CAD build for the part. Positions are in the model's coordinates, mm. A direction names the side the tool comes from. Give positions to 0.01 mm unless a question says otherwise; leave off trailing zeros. Loops run counter-clockwise (first coordinate to the right, second up) from the corner with the lowest first, then second, coordinate; pieces in that order, holes last.
Item 1: Drop flat-ended pins along their axis: P1, Ø2, axis at y = 11.5, z = 5.5, coming from the +X side; P2, Ø6.5, axis at x = -16.5, y = 2.5, coming from the +Z side; P3, Ø1, axis at y = 2, z = 10.5, coming from the +X side; P4, Ø9, axis at x = 18, y = 0, coming from the -Z side. Give the stop position or say it passes through.
Item 2: Saw through at C-C on x = 18. Give the cut face in (y, z), plus the area to 3 significant figures.
Item 3: Saw through at A-A on y = 0. Give the number of separate pieces and of enclosed holes in the cut face, plus the area to 3 significant figures.
Item 4: Saw through at B-B on x = 0. Give the cut face in (y, z).
Item 5: Which spindle directions (+Z, -Z, +X, -X, +Y, -Y) get a long thin tool onto all of the face, cutting with end or side? Do faces 1 (the flat face through (7.02, 8.9, 5.33)), 2 (the flat face through (-5.5, 11, 6)), 3 (the cylindrical face through (20.747, 0.121, 3.328)). Say none if no direction does.
Item 6: Probe probe 1 along X at (y, z) = (0, 4); probe 2 along Z at (x, y) = (-6.6, 10.5); probe 3 along Y at (x, z) = (8, 5.5). List the from-to ranges inside material, lowest first.
Item 7: Mould opens along Y. For faces 4 (the flat face through (7.02, 10.29, 8.47)), 5 (the flat face through (-16.32, -5.74, 3.7)), 6 (the flat face through (23.5, 0, 3)), 7 (the flat face through (7.021, 8.689, 7.304)) say: released by +Y, released by -Y, zero draft, split by the parting line, or undercut.
from build123d import *

# Parameters (mm, degrees)
BOSS_EXTRUDE1_DEPTH                                 = 13
CUT_EXTRUDE1_DEPTH                                  = 24.780243901
CUT_EXTRUDE1_DEPTH_BACK                             = 24.780243901
FILLET1_R                                           = 2
BOSS_EXTRUDE2_DEPTH                                 = 7
F_5_5_5_5_DIAMETER_HOLE1_D                          = 5.5
F_5_5_5_5_DIAMETER_HOLE1_DEPTH                      = 10
F_5_5_5_5_DIAMETER_HOLE1_CSINK_D                    = 6
F_5_5_5_5_DIAMETER_HOLE1_CSINK_ANGLE                = 90
F_5_5_5_5_DIAMETER_HOLE1_TIP                        = 1.652366702
CUT_EXTRUDE2_REACH                                  = 39.017
CBORE_FOR_M4_HEX_SOCKET_HEAD_CAP_SCREW3_D           = 3.4
CBORE_FOR_M4_HEX_SOCKET_HEAD_CAP_SCREW3_CBORE_D     = 7.5
CBORE_FOR_M4_HEX_SOCKET_HEAD_CAP_SCREW3_CBORE_DEPTH = 3
CHAMFER1_SIZE                                       = 0.2
CUT_EXTRUDE3_DEPTH                                  = 3
CHAMFER2_SIZE                                       = 0.5
FILLET2_R                                           = 0.8
CHAMFER3_SIZE                                       = 0.2
CHAMFER3_SIZE2                                      = 0.346410162


with BuildPart() as part:
    # Sketch1 → Boss-Extrude1 (new body)
    with BuildSketch(Plane.XY):
        with BuildLine():
            Line((0.75, 5.95294045), (0.75, 15.5))
            Line((0.75, 15.5), (7.5, 15.5))
            Line((7.5, 15.5), (7.5, 10))
            ThreePointArc((7.5, 10), (0, -12.5), (-7.5, 10))
            Line((-7.5, 10), (-7.5, 15.5))
            Line((-7.5, 15.5), (-0.75, 15.5))
            Line((-0.75, 15.5), (-0.75, 5.95294045))
            ThreePointArc((-0.75, 5.95294045), (0, -6), (0.75, 5.95294045))
        make_face()
    extrude(amount=BOSS_EXTRUDE1_DEPTH)

    # Sketch2 → Cut-Extrude1 (cut, two sides: drawn at the far end of the back side and taken through both)
    with BuildSketch(Plane(origin=(0, 0, 0), x_dir=(0, 0, -1), z_dir=(1, 0, 0)).offset(-CUT_EXTRUDE1_DEPTH_BACK)):
        with BuildLine():
            Line((69.410215856, 1.772448509), (0, 14.891132578))
            ThreePointArc((0, 14.891132578), (-6.5, 15.5), (-13, 14.891132578))
            Line((-13, 14.891132578), (-82.410215856, 1.772448509))
            Line((-82.410215856, 1.772448509), (-82.410215856, 143.050584636))
            Line((-82.410215856, 143.050584636), (69.410215856, 143.050584636))
            Line((69.410215856, 143.050584636), (69.410215856, 1.772448509))
        make_face()
    extrude(amount=CUT_EXTRUDE1_DEPTH + CUT_EXTRUDE1_DEPTH_BACK, mode=Mode.SUBTRACT)

    # Fillet1
    fillet1_edges = [part.edges().sort_by_distance(p)[0] for p in [
        (7.5, 10, 6.5),
        (-7.5, 10, 6.5),
    ]]
    fillet(fillet1_edges, radius=FILLET1_R)

    # Sketch3 → Boss-Extrude2 (add)
    with BuildSketch(Plane.XY):
        with BuildLine():
            Line((8.803538255, 8.873990883), (23.5, 2.75))
            Line((23.5, 2.75), (23.5, -2.75))
            Line((23.5, -2.75), (8.803538255, -8.873990883))
            ThreePointArc((8.803538255, -8.873990883), (12.5, 0), (8.803538255, 8.873990883))
        make_face()
    extrude(amount=BOSS_EXTRUDE2_DEPTH)

    # Mirror1: part across plane


with BuildPart() as part_1:
    add(part.part)
    add(part.part.mirror(Plane(origin=(0, 0, 0), x_dir=(0, 0, 1), z_dir=(1, 0, 0))))

    # Ø5.5 (5.5) Diameter Hole1
    with Locations(Plane.XY.offset(7)):
        with Locations((18, 0), (-18, 0)):
            CounterSinkHole(F_5_5_5_5_DIAMETER_HOLE1_D / 2, F_5_5_5_5_DIAMETER_HOLE1_CSINK_D / 2, depth=F_5_5_5_5_DIAMETER_HOLE1_DEPTH, counter_sink_angle=F_5_5_5_5_DIAMETER_HOLE1_CSINK_ANGLE)
            with Locations((0, 0, -(F_5_5_5_5_DIAMETER_HOLE1_DEPTH + F_5_5_5_5_DIAMETER_HOLE1_TIP / 2))):  # 118° drill point
                Cone(0, F_5_5_5_5_DIAMETER_HOLE1_D / 2, F_5_5_5_5_DIAMETER_HOLE1_TIP, mode=Mode.SUBTRACT)

    # Sketch9 → Cut-Extrude2 (cut, up to next)
    with BuildSketch(Plane(origin=(7.5, 0, 0), x_dir=(0, 0, -1), z_dir=(1, 0, 0)), mode=Mode.PRIVATE) as cut_extrude2_sk1:
        with BuildLine():
            Line((-2.023006126, 10.95445115), (-13, 10.95445115))
            Line((-13, 10.95445115), (-13, 6))
            Line((-13, 6), (-6.5, 6))
            ThreePointArc((-6.5, 6), (-3.161210536, 7.482967532), (-2.023006126, 10.95445115))
        make_face()
    cut_extrude2_tool1 = extrude(cut_extrude2_sk1.sketch, amount=CUT_EXTRUDE2_REACH, mode=Mode.PRIVATE) & part_1.part
    add(cut_extrude2_tool1.solids().sort_by_distance((7.5, 8.604622, 7.889878))[0], mode=Mode.SUBTRACT)

    # CBORE for M4 Hex Socket Head Cap Screw3 (through all)
    with Locations(Plane(origin=(7.5, 0, 0), x_dir=(0, 0, -1), z_dir=(1, 0, 0))):
        with Locations((-6.5, 10.5)):
            CounterBoreHole(CBORE_FOR_M4_HEX_SOCKET_HEAD_CAP_SCREW3_D / 2, CBORE_FOR_M4_HEX_SOCKET_HEAD_CAP_SCREW3_CBORE_D / 2, CBORE_FOR_M4_HEX_SOCKET_HEAD_CAP_SCREW3_CBORE_DEPTH)

    # Sketch12 → Revolve1 (revolve)
    with BuildSketch(Plane.XY.offset(6.5), mode=Mode.PRIVATE) as revolve1_sk:
        Polygon((4.5, 14), (8.5, 14), (8.5, 10.5), (-5.5, 10.5), (-5.5, 12), (-5, 12.5), (4.5, 12.5), align=None)
    revolve(revolve1_sk.sketch.rotate(Axis((0, 10.5, 6.5), (1, 0, 0)), 270), axis=Axis((0, 10.5, 6.5), (1, 0, 0)))

    # Chamfer1
    chamfer1_edges = [part_1.edges().sort_by_distance(p)[0] for p in [
        (8.5, 10.5, 10),
    ]]
    chamfer(chamfer1_edges, length=CHAMFER1_SIZE)

    # Sketch13 → Cut-Extrude3 (cut)
    with BuildSketch(Plane(origin=(8.5, 0, 0), x_dir=(0, 0, -1), z_dir=(1, 0, 0))):
        Polygon((-4.661489956, 11.861177424), (-6.759559206, 12.772785116), (-8.598069251, 11.411607691), (-8.338510044, 9.138822576), (-6.240440794, 8.227214884), (-4.401930749, 9.588392309), align=None)
    extrude(amount=-CUT_EXTRUDE3_DEPTH, mode=Mode.SUBTRACT)

    # Chamfer2
    chamfer2_edges = [part_1.edges().sort_by_distance(p)[0] for p in [
        (-7.5, 12.922791864, 13),
        (-2.211613172, -12.302795096, 13),
        (-7.680564695, 10.123996352, 13),
    ]]
    chamfer(chamfer2_edges, length=CHAMFER2_SIZE)

    # Fillet2
    fillet2_edges = [part_1.edges().sort_by_distance(p)[0] for p in [
        (12.36996926, -1.798293779, 7),
        (8.803538255, -8.873990883, 3.5),
        (-12.5, 0, 7),
        (-8.803538255, -8.873990883, 3.5),
    ]]
    fillet(fillet2_edges, radius=FILLET2_R)

    # Chamfer3
    chamfer3_edges = [part_1.edges().sort_by_distance(p)[0] for p in [
        (0, -6, 13),
    ]]
    chamfer3_side = [part_1.faces().sort_by_distance(p)[0] for p in [
        (0, -6, 6.5),
    ]]
    chamfer(chamfer3_edges, length=CHAMFER3_SIZE, length2=CHAMFER3_SIZE2, reference=chamfer3_side[0])


solid = part_1.part
Results below:
1. P1: stops at x = 8.5
1. P2: stops at z = 7
1. P3: stops at x = 12.41
1. P4: stops at z = 0
2. outline: (-5.04, 0) - (-2.75, 0) - (-2.75, 6.75) - (-3, 7) - (-5.04, 7) - close; (2.75, 0) - (5.04, 0) - (5.04, 7) - (3, 7) - (2.75, 6.75) - close
2. area: 32.0 mm2
3. separate pieces: 4
3. enclosed holes: 0
3. area: 246 mm2
4. outline: (-12.5, 0) - (-6, 0) - (-6, 12.8) - (-6.35, 13) - (-12, 13) - (-12.5, 12.5) - close; circle Ø4 at (10.5, 6.5)
5. face 1: +X
5. face 2: -X
5. face 3: +Z, -Z
6. probe 1: x = -23.5 to -20.75, -15.25 to -6, 6 to 15.25, 20.75 to 23.5
6. probe 2: z = 0 to 4.8, 8.2 to 13
6. probe 3: y = -9.6 to 6.11, 7.15 to 8.78, 12.23 to 13.85
7. face 4: undercut
7. face 5: released by -Y
7. face 6: zero draft
7. face 7: undercut
